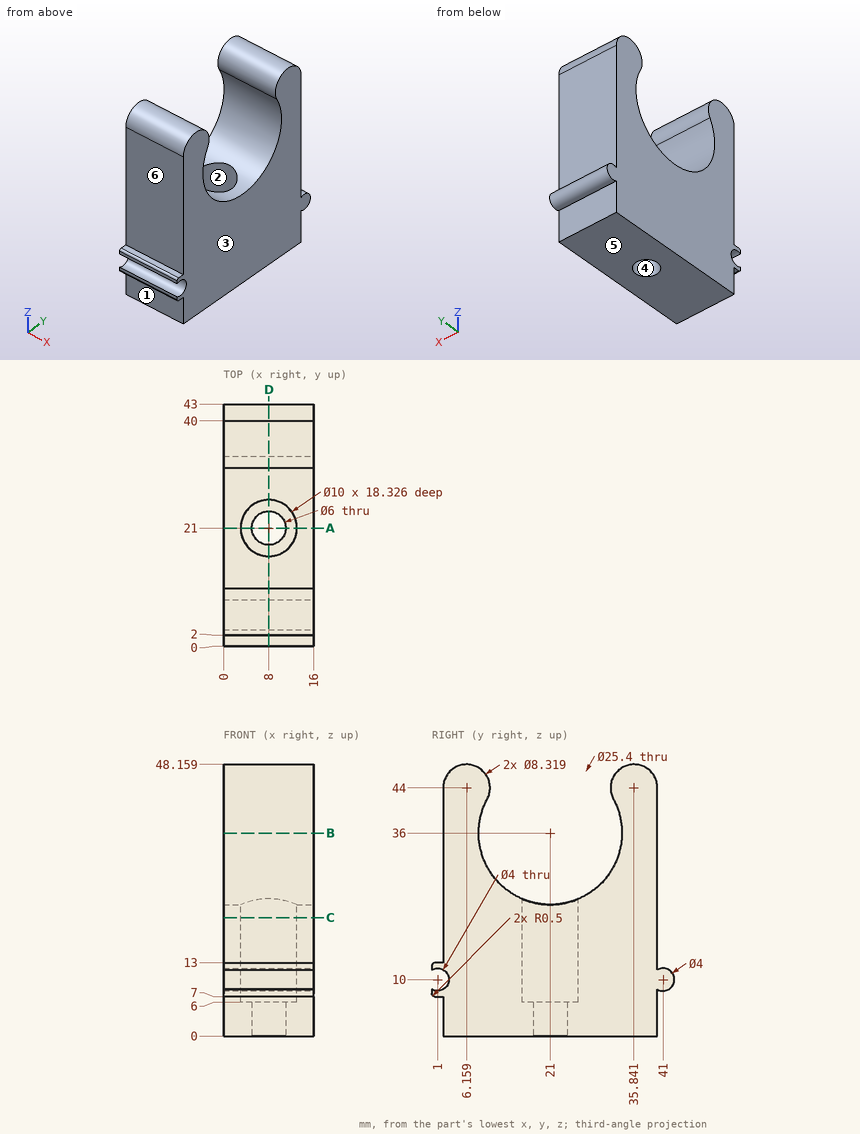
Here's the drawing with two shaded views (mm, measured from the low corner). I have some questions. A direction names the side the tool comes from. Give positions to 0.01 mm unless a question says otherwise; leave off trailing zeros. Order: outer loops, then holes, each group sorted by start corner. A loop starts at its lowest first (then second) coordinate and runs counter-clockwise, first axis right, second up. Notation, with made-up numbers: M 6.5,76 L 61.5,76 A33 cw 61.5,106 Z; hole C 49,44 d3. An arc over 180 degrees is marked long. Answer as a JSON object with one key per item and string values. Group by question number.
1) I'm going to push flat-ended pins straight in: pin 1 Ø2 at (x, z) = (12, 6.5) entering from +Y; pin 2 Ø15 at (y, z) = (21, 36) entering from -X; pin 3 Ø0.8 at (x, y) = (8, 1.5) entering from +Z; pin 4 Ø1.5 at (x, y) = (2.5, 10) entering from +Z (1 decimal). Where does each tip first touch, or does it pass through?
2) We'd pull the mould along X, two halves only. Please class the marked faces 1, 2, 3 and 4: pulls with the +X half, pulls with the -X half, needs draft (parallel to the pull), parting line crosses it, or undercut.
3) Please list where these lines run through material, in increasing order: L1, parallel to Y at x = 6, z = 36; L2, parallel to Y at x = 8, z = 2.1; L3, parallel to Z at x = 10.25, y = 1. Write a range as [from, to].
4) Suppose I cut it at A-A, the plane y = 21. Write out the boundary of the cut face in (x, z).
5) Suppose I cut it at C-C, the plane z = 21. Write out the boundary of the cut face in (x, y).
6) Suppose I cut it at B-B, the plane z = 36. Write out the boundary of the cut face in (x, y), plus the area to 3 significant figures.
7) On a 3-axis mill with a long thin cutter (end or side, diameter ignored), from which of +Z, -Z, +X, -X, +Y, -Y can I reach the whole of each face in a straight line? I mean the marked faces 5 and 6. Say none if no direction works.
8) Suppose I cut it at D-D, the plane x = 8. Write out the boundary of the cut face in (y, z) (1 decimal).
Results found:
{
 "1": {"pin 1": "y = 40", "pin 2": "through", "pin 3": "z = 13", "pin 4": "z = 46.8"},
 "2": {"face 1": "needs draft", "face 2": "undercut", "face 3": "pulls with the +X half", "face 4": "undercut"},
 "3": {"L1": "[2, 8.3], [33.7, 40]", "L2": "[2, 18], [24, 40]", "L3": "[7, 8], [12, 13]"},
 "4": {"outline": "M 0,0 L 5,0 L 5,6 L 3,6 L 3,23.3 L 0,23.3 Z; M 11,0 L 16,0 L 16,23.3 L 13,23.3 L 13,6 L 11,6 Z"},
 "5": {"outline": "M 0,2 L 16,2 L 16,40 L 0,40 Z; hole C 8,21 d10"},
 "6": {"outline": "M 0,2 L 16,2 L 16,8.3 L 0,8.3 Z; M 0,33.7 L 16,33.7 L 16,40 L 0,40 Z", "area": "202 mm²"},
 "7": {"face 5": "-Z, +X, -X, +Y, -Y", "face 6": "+Z, +X, -X, -Y"},
 "8": {"outline": "M 0,7.5 A0.5 ccw 0.5,7 L 2,7 L 2,0 L 18,0 L 18,6 L 16,6 L 16,24.3 A12.7 cw 9.8,42 A4.2 ccw long 2,44 L 2,13 L 0.5,13 A0.5 ccw 0,12.5 L 0,11.7 A2 cw long 0,8.3 Z; M 24,0 L 40,0 L 40,8.3 A2 ccw long 40,11.7 L 40,44 A4.2 ccw long 32.2,42 A12.7 cw 26,24.3 L 26,6 L 24,6 Z"}
}
